Part model, mm, in its own coordinate system. A direction names the side the tool comes from. Round coordinates to 2 decimals unless told otherwise and drop trailing zeros. Loops run counter-clockwise (first coordinate to the right, second up) from the corner with the lowest first, then second, coordinate; pieces in that order, holes last. Notation, with made-up numbers: (6, 24) - (14, 24) arc R32 cw to (14, 54) - close; hole circle Ø1 at (46, 58). An arc over 180 degrees is marked (long way). Write each question's results on one line, items separated by ' | '. Start each with the question number.
(1) Cut at A-A, the plane z = 71. List the corners of the cut face in (x, y), then the cut area to 3 significant figures.
(2) Cut at B-B, the plane x = 9. List the corners of the cut face in (y, z), then the cut area to 3 significant figures.
(3) Cut at D-D, the plane z = 26. List the corners of the cut face in (x, y).
(4) Cut at C-C, the plane y = -12.5. List the corners of the cut face in (x, z), then the cut area to 3 significant figures.
(5) Tool access for faces 1 (the face through (0, -13, 50)), 2 (the face through (10, 0, 50)), 3 (the face through (10.14, -9.812, 45.216)): list every direction of +Z, -Z, +X, -X, +Y, -Y with a clear straight run to the whole face (end or side of a thin tool).
(6) Drill centre lines: L1, parallel to Z at x = 10, y = -12.5; L2, parallel to Z at x = -18.5, y = 41.5; L3, parallel to Y at x = 13, z = 24.5. Where is each one in solid material? Low to high.
(7) Flat gauge pins, fed straight in: P1, Ø6, axis at x = 5.5, z = 41.5, coming from the +Y side; P2, Ø20, axis at y = -17, z = 52.5, coming from the -X side. Where does each tip first touch, or does it go through?
from build123d import *

# Parameters (mm, degrees)
F0_W     = 20
F0_H     = 25
F1_DEPTH = 80
F2_R     = 5
F2_R_2   = 4.5
F3_DEPTH = 25
F4_W     = 20
F4_H     = 20
F5_DEPTH = 72
F6_W     = 97
F6_H     = 20
F7_DEPTH = 55
F8_W     = 75
F8_H     = 97
F9_DEPTH = 80


with BuildPart() as f1:
    # F0 (on Top) → F1 (new body)
    with BuildSketch(Plane.XY):
        with Locations((10, -12.5)):
            Rectangle(F0_W, F0_H)
    extrude(amount=F1_DEPTH)

    # F2 (on face) → F3 (cut)
    with BuildSketch(Plane.YZ.offset(20)):
        with Locations((-12.5, 71)):
            Circle(F2_R)
        with Locations((-12.5, 56)):
            Circle(F2_R_2)
        with Locations((-12.5, 41)):
            Circle(F2_R)
        with Locations((-12.5, 26)):
            Circle(F2_R_2)
    extrude(amount=-F3_DEPTH, mode=Mode.SUBTRACT)

    # F4 (on face) → F5 (join)
    with BuildSketch(Plane(origin=(0, 0, 0), x_dir=(-1, 0, 0), z_dir=(0, 1, 0))):
        with Locations((-10, 10)):
            Rectangle(F4_W, F4_H)
    extrude(amount=F5_DEPTH)

    # F6 (on face) → F7 (join)
    with BuildSketch(Plane(origin=(0, 0, 0), x_dir=(0, -1, 0), z_dir=(-1, 0, 0))):
        with Locations((-23.5, 10)):
            Rectangle(F6_W, F6_H)
    extrude(amount=F7_DEPTH)

    # F8 (on face) → F9 (join)
    with BuildSketch(Plane(origin=(0, 0, 0), x_dir=(1, 0, 0), z_dir=(0, 0, -1))):
        with Locations((-17.5, -23.5)):
            Rectangle(F8_W, F8_H)
    extrude(amount=F9_DEPTH)


solid = f1.part
A:
1) outline: (0, -25) - (20, -25) - (20, -17.5) - (0, -17.5) - close; (0, -7.5) - (20, -7.5) - (20, 0) - (0, 0) - close | area: 300 mm2
2) outline: (-25, -80) - (72, -80) - (72, 20) - (0, 20) - (0, 80) - (-25, 80) - close; hole circle Ø10 at (-12.5, 41); hole circle Ø10 at (-12.5, 71); hole circle Ø9 at (-12.5, 26); hole circle Ø9 at (-12.5, 56) | area: 10,900 mm2
3) outline: (0, -25) - (20, -25) - (20, -17) - (0, -17) - close; (0, -8) - (20, -8) - (20, 0) - (0, 0) - close
4) outline: (-55, -80) - (20, -80) - (20, 21.5) - (0, 21.5) - (0, 20) - (-55, 20) - close; (0, 30.5) - (20, 30.5) - (20, 36) - (0, 36) - close; (0, 46) - (20, 46) - (20, 51.5) - (0, 51.5) - close; (0, 60.5) - (20, 60.5) - (20, 66) - (0, 66) - close; (0, 76) - (20, 76) - (20, 80) - (0, 80) - close | area: 7,940 mm2
5) face 1: +Z, -X, +Y, -Y | face 2: +Z, +X, -X, +Y | face 3: +X, -X
6) L1: -80 to 21.5, 30.5 to 36, 46 to 51.5, 60.5 to 66, 76 to 80 | L2: -80 to 20 | L3: -25 to -16.74, -8.26 to 0
7) P1: y = 0 | P2: x = 0
